```python
from build123d import *

# Parameters (mm, degrees)
ESBO_O2_R                = 12.5
ESBO_O2_R_2              = 10.5
RESSALTO_EXTRUS_O1_DEPTH = 230.5
ESBO_O3_W                = 2
ESBO_O3_H                = 5
CORTE_EXTRUS_O1_DEPTH    = 60


with BuildPart() as part:
    # Esboço2 → Ressalto-extrusão1 (new, symmetric)
    with BuildSketch(Plane(origin=(0, 0, 0), x_dir=(0, 0, -1), z_dir=(1, 0, 0))):
        Circle(ESBO_O2_R)
        Circle(ESBO_O2_R_2, mode=Mode.SUBTRACT)
    extrude(amount=RESSALTO_EXTRUS_O1_DEPTH, both=True)

    # Esboço3 → Corte-extrusão1 (cut)
    with BuildSketch(Plane(origin=(230.5, 0, 0), x_dir=(0, 0, -1), z_dir=(1, 0, 0))):
        with Locations((0, 12.5)):
            Rectangle(ESBO_O3_W, ESBO_O3_H)
    corte_extrus_o1 = extrude(amount=-CORTE_EXTRUS_O1_DEPTH, mode=Mode.SUBTRACT)

    # Espelhar1: Corte-extrusão1 across plane
    add(corte_extrus_o1.mirror(Plane(origin=(0, 0, 0), x_dir=(0, 0, 1), z_dir=(1, 0, 0))), mode=Mode.SUBTRACT)


solid = part.part
```
Check sheet for the modelled part. Datum: model origin and axes. Units: mm. Give positions to 0.01 mm unless a question says otherwise; leave off trailing zeros. Loops run counter-clockwise (first coordinate to the right, second up) from the corner with the lowest first, then second, coordinate; pieces in that order, holes last. Notation, with made-up numbers: M -40,86.5 L -35,86.5 A20 ccw -35,108.5 Z; hole C 85.5,-15.5 d11. An arc over 180 degrees is marked long. Answer as CSV lines item,"result".
Item 1: Draft check along Y on faces 1 (the face through (-3.2, 3.2, -10)), 2 (the face through (-230.5, -9, 6)), 3 (the face through (3.227, 3.755, -11.923)). Enter one of: pulls with the +Y half, pulls with the -Y half, needs draft (parallel to the pull), parting line crosses it, or undercut.
Reply:
face 1,"undercut"
face 2,"needs draft"
face 3,"parting line crosses it"
Item 2: Sectioned sample at A-A, the plane y = 0. Enter the section's corners in (x, z), then the cut area to 3 significant figures.
Reply:
outline,"M -230.5,-12.5 L 230.5,-12.5 L 230.5,-10.5 L -230.5,-10.5 Z; M -230.5,10.5 L 230.5,10.5 L 230.5,12.5 L -230.5,12.5 Z"
area,"1,840 mm^2"
Item 3: Sectioned sample at C-C, the plane z = -6. Enter the section's corners in (x, y), then the cut area to 3 significant figures.
Reply:
outline,"M -230.5,-10.97 L 230.5,-10.97 L 230.5,-8.62 L -230.5,-8.62 Z; M -230.5,8.62 L 230.5,8.62 L 230.5,10.97 L -230.5,10.97 Z"
area,"2,170 mm^2"
Item 4: Scan lines: L1, parallel to Z at x = 25.5, y = 0; L2, parallel to Y at x = 31, z = -2. Record each from-to range of solid material in increasing order.
Reply:
L1,"-12.5 to -10.5, 10.5 to 12.5"
L2,"-12.34 to -10.31, 10.31 to 12.34"
Item 5: Depth check by flat-ended pin: pin 1 Ø1 at (x, y) = (-109.5, 1.5) entering from -Z; pin 2 Ø8 at (x, z) = (-179.5, 5.5) entering from -Y; pin 3 Ø3 at (x, y) = (-105, -5.5) entering from +Z. Enter the tip coordinate at first touch or a pass-through.
Reply:
pin 1,"z = -12.46"
pin 2,"y = -12.41"
pin 3,"z = 11.84"
Item 6: Sectioned sample at D-D, the plane x = -201. Enter the section's corners in (y, z), then the cut area to 3 significant figures.
Reply:
outline,"M 10.45,-1 A10.5 cw long 10.45,1 L 12.46,1 A12.5 ccw long 12.46,-1 Z"
area,"141 mm^2"
Item 7: Sectioned sample at B-B, the plane x = -88. Enter the section's corners in (y, z).
Reply:
outline,"C 0,0 d25; hole C 0,0 d21"
